Design review of the part built by this model. Coordinates are the model's own, in mm. Face numbers are marked on the shaded views. A direction names the side the tool comes from. Give positions to 0.01 mm unless a question says otherwise; leave off trailing zeros. Loops run counter-clockwise (first coordinate to the right, second up) from the corner with the lowest first, then second, coordinate; pieces in that order, holes last. Notation, with made-up numbers: M -14,71.25 L 3,71.25 A32 ccw 3,107.25 Z; hole C 0,1 d2. An arc over 180 degrees is marked long. Use CSV: the item, a comma, the result in double quotes.
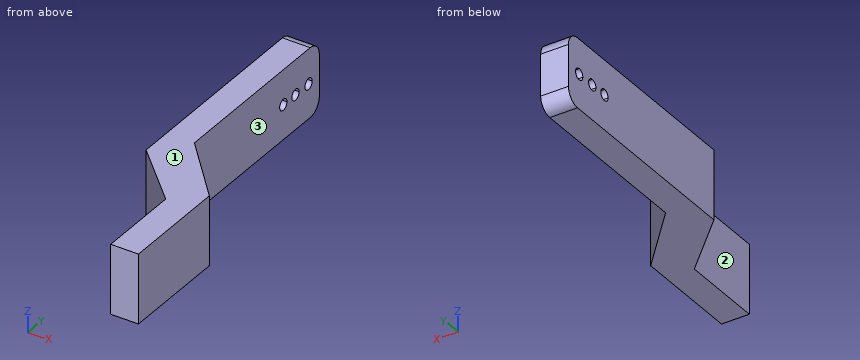
from build123d import *

# Parameters (mm, degrees)
Y_KSEKLIK_EKSTR_ZYON1_DEPTH = 25
KES_EKSTR_ZYON1_DEPTH       = 25
RADYUS1_R                   = 5
RADYUS2_R                   = 5


with BuildPart() as part:
    # Çizim1 → Yükseklik-Ekstrüzyon1 (new body)
    with BuildSketch(Plane.XY):
        Polygon((30, -11.002799306), (30, -50), (20, -50), (20, -19.736164581), (0, 0), (0, 80), (10, 80), (10, 11.297306062), align=None)
    extrude(amount=Y_KSEKLIK_EKSTR_ZYON1_DEPTH)

    # Çizim2 → Kes-Ekstrüzyon1 (cut)
    with BuildSketch(Plane.ZY):
        with BuildLine():
            ThreePointArc((14.5, 74.088859677), (13.914213562, 75.50307324), (12.5, 76.088859677))
            Line((12.5, 76.088859677), (12.5, 72.088859677))
            ThreePointArc((12.5, 72.088859677), (13.914213562, 72.674646115), (14.5, 74.088859677))
        make_face()
        with BuildLine():
            Line((12.5, 72.088859677), (12.5, 76.088859677))
            ThreePointArc((12.5, 76.088859677), (10.5, 74.088859677), (12.5, 72.088859677))
        make_face()
        with BuildLine():
            ThreePointArc((14.5, 66.903895924), (13.914213562, 68.318109486), (12.5, 68.903895924))
            Line((12.5, 68.903895924), (12.5, 64.903895924))
            ThreePointArc((12.5, 64.903895924), (13.914213562, 65.489682361), (14.5, 66.903895924))
        make_face()
        with BuildLine():
            Line((12.5, 64.903895924), (12.5, 68.903895924))
            ThreePointArc((12.5, 68.903895924), (10.5, 66.903895924), (12.5, 64.903895924))
        make_face()
        with BuildLine():
            ThreePointArc((12.5, 62.207705215), (10.5, 60.207705215), (12.5, 58.207705215))
            Line((12.5, 58.207705215), (12.5, 62.207705215))
        make_face()
        with BuildLine():
            Line((12.5, 62.207705215), (12.5, 58.207705215))
            ThreePointArc((12.5, 58.207705215), (13.914213562, 58.793491652), (14.5, 60.207705215))
            ThreePointArc((14.5, 60.207705215), (13.914213562, 61.621918777), (12.5, 62.207705215))
        make_face()
    extrude(amount=-KES_EKSTR_ZYON1_DEPTH, mode=Mode.SUBTRACT)

    # Radyus1
    radyus1_edges = [part.edges().sort_by_distance(p)[0] for p in [
        (5, 80, 25),
    ]]
    fillet(radyus1_edges, radius=RADYUS1_R)

    # Radyus2
    radyus2_edges = [part.edges().sort_by_distance(p)[0] for p in [
        (5, 80, 0),
    ]]
    fillet(radyus2_edges, radius=RADYUS2_R)


solid = part.part
(1) We need section C-C on y = 24.5. State the section outline as (x, z) points.
A:
outline,"M 0,0 L 10,0 L 10,25 L 0,25 Z"
(2) We need section A-A on x = 5.75. State the section outline as (y, z) points, then the cut area to 3 significant figures.
A:
outline,"M -5.67,0 L 75,0 A5 ccw 80,5 L 80,20 A5 ccw 75,25 L -5.67,25 Z; hole C 60.21,12.5 d4; hole C 66.9,12.5 d4; hole C 74.09,12.5 d4"
area,"2,090 mm²"
(3) We need section D-D on x = 16.25. State the section outline as (y, z) points.
A:
outline,"M -16.04,0 L 4.33,0 L 4.33,25 L -16.04,25 Z"
(4) Wall thickness on line 1 along X through (y, z) = (71, 8.5); line 2 along X through (y, z) = (-26.5, 19.75); line 3 along Z through (x, y) = (7, 66): over which ranges is each line inside the solid? List them lowest first. Write a range as [from, to].
A:
line 1,"[0, 10]"
line 2,"[20, 30]"
line 3,"[0, 10.72], [14.28, 25]"
(5) Clearance check with flat-ended pins moving along their axes: P1, Ø4, axis at y = 9, z = 12.5, coming from the -X side; P2, Ø12.5, axis at y = -36.5, z = 12, coming from the -X side; P3, Ø5, axis at x = 25, z = 14, coming from the +Y side; P4, Ø2, axis at y = 40, z = 14, coming from the +X side. State where each tip first meets the part, or that it passes through.
A:
P1,"x = 0"
P2,"x = 20"
P3,"y = -2.64"
P4,"x = 10"
(6) Machinability: for the marked faces 1, 2 and 3, which of the approach directions +Z, -Z, +X, -X, +Y, -Y give a long, thin tool a straight path to every point of the face, cutting with its end or side? Answer none if there is none.
A:
face 1,"+Z, +X, -X, +Y, -Y"
face 2,"+Z, -Z, -X, -Y"
face 3,"+Z, -Z, +X, +Y"
(7) We need section B-B on z = 16. State the section outline as (x, y) points.
A:
outline,"M 0,0 L 20,-19.74 L 20,-50 L 30,-50 L 30,-11 L 10,11.3 L 10,80 L 0,80 Z"
